For this review, take the finished solid that the model builds, in its own axes (mm). Face numbers are marked on the shaded views. A direction names the side the tool comes from. Give positions to 0.01 mm unless a question says otherwise; leave off trailing zeros. Loops run counter-clockwise (first coordinate to the right, second up) from the corner with the lowest first, then second, coordinate; pieces in that order, holes last.
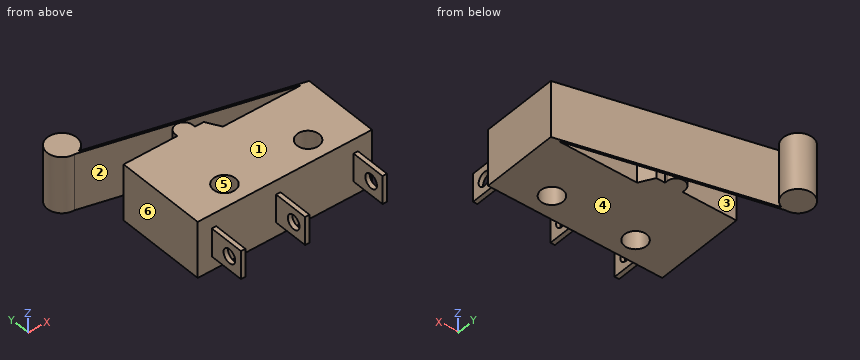
Autodesk Inventor part; units mm, degrees
ref_plane "YZ Plane" through (0, 0, 0) normal (1, 0, 0) x (0, 1, 0)
ref_plane "XZ Plane" through (0, 0, 0) normal (0, 1, 0) x (-1, 0, 0)
ref_plane "XY Plane" through (0, 0, 0) normal (0, 0, 1) x (1, 0, 0)
sketch "Sketch1" plane through (0, 0, 0) normal (0, 0, 1) x (1, 0, 0)
  line L0 (0, 0) -> (0, 10.2)
  line L1 (0, 10.2) -> (9.1, 10.2)
  line L2 (9.1, 10.2) -> (9.99, 8.6487)
  line L3 (9.99, 8.6487) -> (19.8, 8.6487)
  line L4 (19.8, 8.6487) -> (19.8, 0)
  line L5 (19.8, 0) -> (0, 0)
  circle A0 centre (5.1, 2.5) radius 1.25
  circle A1 centre (14.6, 2.5) radius 1.25
  arc A2 (8.1, 10.5) -> (6.1001, 10.4874) centre (7.1, 10.5) ccw
  line L6 (8.1, 10.5) -> (8.1, 10.2)
  line L7 (6.1001, 10.5) -> (6.1001, 10.2)
  dimension "d0" = 9.1
  dimension "d1" = 10.2
  dimension "d2" = 19.8
  dimension "d3" = 2.5
  dimension "d4" = 5.1
  dimension "d5" = 2.5
  dimension "d6" = 9.5
  dimension "d7" = 2.5
  dimension "d8" = 2.5
  dimension "d9" = 2
  dimension "d10" = 7.5
  dimension "d11" = 10.5
extrude "Extrusion1" add sketch "Sketch1" along normal blind 6.4
sketch "Sketch3" plane through (0, 0, 0) normal (0, -1, 0) x (1, 0, 0)
  line L0 (8.9, 1.6) -> (8.9, 4.8)
  line L1 (8.9, 4.8) -> (9.4, 4.8)
  line L2 (9.4, 4.8) -> (9.4, 1.6)
  line L3 (9.4, 1.6) -> (8.9, 1.6)
  line L4 (17.7, 1.6) -> (17.7, 4.8)
  line L5 (17.7, 4.8) -> (18.2, 4.8)
  line L6 (18.2, 4.8) -> (18.2, 1.6)
  line L7 (18.2, 1.6) -> (17.7, 1.6)
  line L8 (1.6, 1.6) -> (1.6, 4.8)
  line L9 (1.6, 4.8) -> (2.1, 4.8)
  line L10 (2.1, 4.8) -> (2.1, 1.6)
  line L11 (2.1, 1.6) -> (1.6, 1.6)
extrude "Extrusion3" add sketch "Sketch3" along normal blind 4
sketch "Sketch4" plane through (18.2, 0, 4.8) normal (1, 0, 0) x (0, 0, -1)
  circle A0 centre (1.6, -2.4215) radius 0.8
  point P0 (4.8, 0)
  dimension "d24" = 1.6
extrude "Extrusion4" cut sketch "Sketch4" against normal blind 22
sketch "Sketch5" plane through (0, 0, 6.4) normal (0, 0, 1) x (1, 0, 0)
  line L0 (19.8, 8.6487) -> (9.99, 8.6487)
  line L1 (18.8606, 8.6487) -> (-2.9473, 14.1382)
  line L2 (-2.9473, 14.1382) -> (-2.4872, 14.2588)
  line L3 (-2.4872, 14.2588) -> (19.8, 8.6487)
  circle A0 centre (-2.4872, 15.6717) radius 1.6664
extrude "Extrusion5" add sketch "Sketch5" against normal blind 6.4
sketch "Sketch2" plane through (0, 0, 6.4) normal (0, 0, 1) x (1, 0, 0)
  line L0 (1.6916, 0) -> (2.1916, 0)
  line L1 (2.1916, 0) -> (2.1916, -4)
  line L2 (2.1916, -4) -> (1.6916, -4)
  line L3 (1.6916, -4) -> (1.6916, 0)
  line L4 (10.4916, 0) -> (10.9916, 0)
  line L5 (10.9916, 0) -> (10.9916, -4)
  line L6 (10.9916, -4) -> (10.4916, -4)
  line L7 (10.4916, -4) -> (10.4916, 0)
  line L8 (17.7916, 0) -> (18.2916, 0)
  line L9 (18.2916, 0) -> (18.2916, -4)
  line L10 (18.2916, -4) -> (17.7916, -4)
  line L11 (17.7916, -4) -> (17.7916, 0)
  point P0 (0, 0)
  point P1 (-19.8, 0)
  dimension "d14" = 0.5
  dimension "d15" = 4
  dimension "d16" = 0.5
  dimension "d17" = 0.5
  dimension "d18" = 8.3
  dimension "d19" = 6.8
properties part number "endstopLever"
Q1. Consider section D-D on x = 14.6. Give the boundary of the cut face in (y, z), plus the area to 3 significant figures.
Answers:
outline: (0, 0) - (1.25, 0) - (1.25, 6.4) - (0, 6.4) - close; (3.75, 0) - (8.65, 0) - (8.65, 6.4) - (3.75, 6.4) - close; (9.72, 0) - (9.96, 0) - (9.96, 6.4) - (9.72, 6.4) - close
area: 40.9 mm2
Q2. Consider section A-A on y = 2.5. Give the boundary of the cut face in (x, z).
Answers:
outline: (0, 0) - (3.85, 0) - (3.85, 6.4) - (0, 6.4) - close; (6.35, 0) - (13.35, 0) - (13.35, 6.4) - (6.35, 6.4) - close; (15.85, 0) - (19.8, 0) - (19.8, 6.4) - (15.85, 6.4) - close
Q3. For probe 1 along Y at (x, z) = (17.85, 3.2); probe 2 along Y at (x, z) = (4.25, 2.25); probe 3 along X at (y, z) = (2, 4), list the stretches that pass through material, from the lowest coordinate up.
Answers:
probe 1: y = -4 to -3.22, -1.62 to 8.65, 8.9 to 9.14
probe 2: y = 0 to 1.58, 3.42 to 10.2, 12.33 to 12.56
probe 3: x = 0 to 3.95, 6.25 to 13.45, 15.75 to 19.8
Q4. Mouldability with a two-part tool opening along X and no side actions: class the marked faces 4, 5 and 6 as +X half, -X half, draft (parallel to the pull), parting line (faces both ways), or undercut.
Answers:
face 4: draft
face 5: undercut
face 6: -X half
Q5. Consider section C-C on z = 3.2. Count the separate pieces of the cut face and the enclosed holes in it, plus the area to 3 significant figures.
Answers:
separate pieces: 4
enclosed holes: 2
area: 196 mm2
Q6. Machinability: for the marked faces 1, 2 and 3, which of the approach directions +Z, -Z, +X, -X, +Y, -Y give a long, thin tool a straight path to every point of the face, cutting with its end or side? Answer none if there is none.
Answers:
face 1: +Z, +X, -X, +Y, -Y
face 2: +Z, -Z
face 3: +Z, -Z, -X
Q7. For pin 1 Ø0.6 at (x, y) = (18, -2) entering from +Z; pin 2 Ø1.8 at (x, z) = (2, 2) entering from +Y; pin 3 Ø2 at (y, z) = (-2.42, 3.2) entering from -X, all flat-tipped, find the tip position at first contact; note any pin that passes through.
Answers:
pin 1: stops at z = 4.8
pin 2: stops at y = 13.36
pin 3: stops at x = 1.6
Q8. Consider section B-B on z = 6. Give the boundary of the cut face in (x, y), plus the area to 3 significant figures.
Answers:
outline: (-2.42, 14.01) - (18.86, 8.65) - (9.99, 8.65) - (9.1, 10.2) - (8.1, 10.2) - (8.1, 10.5) arc R1 ccw (long way) to (6.1, 10.49) - (6.1, 10.2) - (0, 10.2) - (0, 0) - (19.8, 0) - (19.8, 8.65) - (-1.9, 14.11) arc R1.67 ccw (long way) to start; hole circle Ø2.5 at (5.1, 2.5); hole circle Ø2.5 at (14.6, 2.5)
area: 192 mm2
